Part model, mm, in its own coordinate system. Coordinates: 2 decimals unless noted, no trailing zeros. Write each loop counter-clockwise with the first axis right and the second up, starting at its lowest first coordinate (ties: lowest second). Pieces come first, ordered by that corner, then holes. Notation, with made-up numbers: (-14.75, 51.25) -> (38.25, 51.25) arc R26 ccw to (38.25, 78.25) -> close; hole circle Ø10 at (-33.75, 18). An arc over 180 degrees is marked (long way). Write item = value, one per line.
from build123d import *

# Parameters (mm, degrees)
F2_R = 5.08


with BuildPart() as f1:
    # F0 (on Front) → F1 (revolve)
    with BuildSketch(Plane.XZ):
        with BuildLine():
            Line((0, 6.7818), (0, 0))
            Line((0, 0), (30.0609, 0))
            Line((30.0609, 0), (44.062068, 145.664361))
            ThreePointArc((44.062068, 145.664361), (42.726161, 147.310607), (41.0591, 146.000767))
            Line((41.0591, 146.000767), (23.241, 6.7818))
            Line((23.241, 6.7818), (0, 6.7818))
        make_face()
    revolve(axis=Axis((0, 0, 3.3909), (0, 0, -1)))

    # F2
    f2_edges = [f1.edges().sort_by_distance(p)[0] for p in [
        (-30.0609, 0, 0),
        (-23.241, 0, 6.7818),
    ]]
    fillet(f2_edges, radius=F2_R)


solid = f1.part
Q1. Mould opens along X. For faces 1 (the face through (0, 0, 6.782)), 2 (the face through (0, 0, 0)), 3 (the face through (-4.87, -37.06, 76.12)) say: released by +X, released by -X, zero draft, split by the parting line, or undercut.
Model answer:
face_1 = undercut
face_2 = zero draft
face_3 = split by the parting line
Q2. Saw through at A-A on y = 0. Give the cut face in (x, z).
Model answer:
outline = (-44.06, 145.66) -> (-30.5, 4.59) arc R5.08 ccw to (-25.45, 0) -> (25.45, 0) arc R5.08 ccw to (30.5, 4.59) -> (44.06, 145.66) arc R1.51 ccw to (41.06, 146) -> (23.81, 11.22) arc R5.08 cw to (18.77, 6.78) -> (-18.77, 6.78) arc R5.08 cw to (-23.81, 11.22) -> (-41.06, 146) arc R1.51 ccw to start
Q3. Probe line 1 (Y direction, x = 23, z = 18); line 2 (Y direction, x = 11, z = 79.5); line 3 (X direction, y = 3, z = 101.5). List the from-to ranges inside material, lowest first. Write a range as from..to.
Model answer:
line_1 = -21.95..-8.94, 8.94..21.95
line_2 = -36.06..-30.63, 30.63..36.06
line_3 = -39.7..-35.24, 35.24..39.7
Q4. Saw through at D-D on z = 86.5. Give the cut face in (x, y), and give its area (3 significant figures).
Model answer:
outline = circle Ø76.75 at (0, 0); hole circle Ø66.89 at (0, 0)
area = 1,110 mm²
Q5. Pin check, flat tips, straight feed: pin 1 (4 mm diameter, centred on x = -14.5, z = 43.5, fed in from +Y); pin 2 (1 mm diameter, centred on x = -30.5, z = 59.5, fed in from +Y); pin 3 (4 mm diameter, centred on y = 10, z = 74, fed in from +X). Stop position of each tip, or through.
Model answer:
pin_1 = 31.91
pin_2 = 19.5
pin_3 = 36.34
Q6. Saw through at C-C on z = 70. Give the cut face in (x, y), and give its area (3 significant figures).
Model answer:
outline = circle Ø73.58 at (0, 0); hole circle Ø62.66 at (0, 0)
area = 1,170 mm²
